```python
from build123d import *

# Parameters (mm, degrees)
F0_W     = 3.175
F0_H     = 35
F1_DEPTH = 3.175


with BuildPart() as f1:
    # F0 (on Top) → F1 (new body)
    with BuildSketch(Plane.XY):
        Polygon((137.5, 0), (162.5, 0), (187.5, 0), (187.5, -3.175), (300, -3.175), (300, 0), (325, 0), (325, 20), (328.175, 20), (328.175, 55), (325, 55), (325, 95), (328.175, 95), (328.175, 130), (325, 130), (325, 150), (300, 150), (300, 153.175), (187.5, 153.175), (187.5, 150), (162.5, 150), (137.5, 150), (137.5, 153.175), (25, 153.175), (25, 150), (0, 150), (0, 130), (-3.175, 130), (-3.175, 95), (0, 95), (0, 55), (-3.175, 55), (-3.175, 20), (0, 20), (0, 0), (25, 0), (25, -3.175), (137.5, -3.175), align=None)
        with Locations((301.5875, 37.5)):
            Rectangle(F0_W, F0_H, mode=Mode.SUBTRACT)
        with Locations((301.5875, 112.5)):
            Rectangle(F0_W, F0_H, mode=Mode.SUBTRACT)
    extrude(amount=F1_DEPTH)


solid = f1.part
```
Could you check a few things on this model? Use its own coordinates, in mm. Round coordinates to 2 decimals unless told otherwise and drop trailing zeros. Loops run counter-clockwise (first coordinate to the right, second up) from the corner with the lowest first, then second, coordinate; pieces in that order, holes last. Notation, with made-up numbers: (63, 80.5) - (111, 80.5) arc R23 cw to (111, 105.5) - close; hole circle Ø8 at (9, -34). An arc over 180 degrees is marked (long way). Answer in a Markdown table with one row per item. Add a question column.
(1) If we section it at B-B (x = 179): Please give me the cut outline in (y, z) (3 decimals), plus the area to 3 significant figures.
(2) I need wall thicknesses on line 1 along X through (y, z) = (102.5, 2.85) (3 decimals); line 2 along X through (y, z) = (94, 2.3); line 3 along Y through (x, z) = (172, 1.4). Which ranges of each line are inside material? Lowest first, please.
(3) If we section it at A-A (z = 1.3): State how many separate pieces and enclosed holes the cut face has, plus the area to 3 significant figures.
(4) If we section it at C-C (y = 11.5): Please give me the cut outline in (x, z) (3 decimals).
(5) I'm going to push flat-ended pins straight in: pin 1 (1.6 mm diameter, centred on x = 326.5, z = 2, fed in from +Y); pin 2 (3 mm diameter, centred on x = 141, y = 102, fed in from -Z); pin 3 (1 mm diameter, centred on y = 15, z = 2, fed in from +X); pin 4 (1.6 mm diameter, centred on x = 308.5, z = 1, fed in from +Y). Where does each tip first touch, or does it pass through?
Model answer:
| question | item | result |
|---|---|---|
| 1 | outline | (0, 0) - (150, 0) - (150, 3.175) - (0, 3.175) - close |
| 1 | area | 476 mm² |
| 2 | line 1 | x = -3.175 to 300, 303.175 to 328.175 |
| 2 | line 2 | x = 0 to 325 |
| 2 | line 3 | y = 0 to 150 |
| 3 | separate pieces | 1 |
| 3 | enclosed holes | 2 |
| 3 | area | 50,400 mm² |
| 4 | outline | (0, 0) - (325, 0) - (325, 3.175) - (0, 3.175) - close |
| 5 | pin 1 | stops at y = 130 |
| 5 | pin 2 | stops at z = 0 |
| 5 | pin 3 | stops at x = 325 |
| 5 | pin 4 | stops at y = 150 |
